Autodesk Inventor part; units mm, degrees
ref_plane "YZ Plane" through (0, 0, 0) normal (1, 0, 0) x (0, 1, 0)
ref_plane "XZ Plane" through (0, 0, 0) normal (0, 1, 0) x (-1, 0, 0)
ref_plane "XY Plane" through (0, 0, 0) normal (0, 0, 1) x (1, 0, 0)
sketch "Sketch1" plane through (0, 0, 0) normal (1, 0, 0) x (0, 1, 0)
  line L0 (10.2141, 17.9541) -> (-31.7859, 17.9541)
  line L1 (-31.7859, 17.9541) -> (-31.7859, -30.1559)
  line L2 (-31.7859, -30.1559) -> (10.2141, -30.1559)
  line L3 (10.2141, -30.1559) -> (10.2141, 17.9541)
  point P0 (0, 0)
  dimension "d0" = 42
  dimension "d1" = 48.11
extrude "BasePlate" add sketch "Sketch1" along normal blind 3
sketch "Sketch2" plane through (3, 0, 0) normal (1, 0, 0) x (0, 0, -1)
  point P0 (0, 0)
sketch "Sketch3" plane through (3, 0, 0) normal (1, 0, 0) x (0, 0, -1)
  line L0 (30.1559, 10.2141) -> (-17.9541, 10.2141)
  line L1 (-17.9541, -31.7859) -> (30.1559, -31.7859)
  line L2 (-17.9541, 10.2141) -> (30.1559, 10.2141)
  line L3 (30.1559, 10.2141) -> (30.1559, -31.7859)
  line L4 (30.1559, -31.7859) -> (-17.9541, -31.7859)
  line L5 (-17.9541, -31.7859) -> (-17.9541, 10.2141)
  line L6 (-15.5541, 8.2141) -> (27.7559, 8.2141)
  line L7 (27.7559, 8.2141) -> (27.7559, -29.3859)
  line L8 (27.7559, -29.3859) -> (-15.5541, -29.3859)
  line L9 (-15.5541, -29.3859) -> (-15.5541, 8.2141)
  point P0 (0, 0)
  point P1 (-17.9541, -10.7859)
  dimension "d4" = 2
  dimension "d5" = 2.4
  dimension "d6" = 2.4
  dimension "d7" = 2.4
extrude "Walls" add sketch "Sketch3" along normal blind 18.5
sketch "Sketch4" plane through (21.5, 0, 0) normal (1, 0, 0) x (0, 0, -1)
  line L0 (30.1559, 10.2141) -> (-17.9541, 10.2141)
  line L1 (-15.5541, 8.2141) -> (27.7559, 8.2141)
  line L2 (-4.1541, 10.2141) -> (5.2459, 10.2141)
  line L3 (5.2459, 10.2141) -> (5.2459, 8.2141)
  line L4 (5.2459, 8.2141) -> (-4.1541, 8.2141)
  line L5 (-4.1541, 8.2141) -> (-4.1541, 10.2141)
  line L6 (-17.9541, 10.2141) -> (-17.9541, -31.7859)
  point P0 (0, 0)
  point P1 (-4.1541, 9.2141)
  point P2 (5.2459, 10.2141)
  dimension "d10" = 9.4
  dimension "d11" = 13.8
extrude "USB-C" cut sketch "Sketch4" against normal blind 10.1
sketch "Sketch5" plane through (21.5, 0, 0) normal (1, 0, 0) x (0, 0, -1)
  line L0 (-17.9541, 10.2141) -> (-17.9541, -31.7859)
  line L1 (-15.5541, -29.3859) -> (-15.5541, 8.2141)
  line L2 (-17.9541, -4.8859) -> (-15.5541, -4.8859)
  line L3 (-15.5541, -4.8859) -> (-15.5541, 7.5141)
  line L4 (-15.5541, 7.5141) -> (-17.9541, 7.5141)
  line L5 (-17.9541, 7.5141) -> (-17.9541, -4.8859)
  line L6 (-4.1541, 10.2141) -> (-17.9541, 10.2141)
  point P0 (0, 0)
  point P1 (-16.7541, 7.5141)
  point P2 (-17.9541, 7.5141)
  point P3 (-15.5541, -4.8859)
  dimension "d14" = 12.4
  dimension "d15" = 2.7
extrude "PowerConnector1" cut sketch "Sketch5" against normal blind 15.5
sketch "Sketch6" plane through (6, 0, 0) normal (1, 0, 0) x (0, 0, -1)
  line L0 (-17.9541, 10.2141) -> (-17.9541, -31.7859)
  line L1 (-17.9541, -0.3859) -> (-15.5541, -0.3859)
  line L2 (-15.5541, -0.3859) -> (-15.5541, 1.6141)
  line L3 (-15.5541, 1.6141) -> (-17.9541, 1.6141)
  line L4 (-17.9541, 1.6141) -> (-17.9541, -0.3859)
  line L5 (-17.9541, 7.5141) -> (-15.5541, 7.5141)
  point P0 (0, 0)
  dimension "d18" = 2.4
  dimension "d19" = 2
  dimension "d20" = 5.9
extrude "PowerConnector2" cut sketch "Sketch6" against normal blind 2.5
sketch "Sketch8" plane through (21.5, 0, 0) normal (1, 0, 0) x (0, 0, -1)
  line L0 (-17.9541, 10.2141) -> (-17.9541, -31.7859)
  line L1 (-15.5541, 8.2141) -> (-15.5541, -29.3859)
  line L2 (-17.9541, -28.7859) -> (-15.5541, -28.7859)
  line L3 (-15.5541, -28.7859) -> (-15.5541, -15.1859)
  line L4 (-15.5541, -15.1859) -> (-17.9541, -15.1859)
  line L5 (-17.9541, -15.1859) -> (-17.9541, -28.7859)
  line L6 (-17.9541, -31.7859) -> (30.1559, -31.7859)
  point P0 (0, 0)
  dimension "d23" = 13.6
  dimension "d24" = 3
extrude "RJ-12" cut sketch "Sketch8" against normal blind 18.1
fillet "Fillet1" radius 0.5 4 edges at (10.75, 10.2141, 17.9541) (10.75, -31.7859, 17.9541) (10.75, 10.2141, -30.1559) (10.75, -31.7859, -30.1559)
sketch "Sketch9" plane through (0, 0, 0) normal (-1, 0, 0) x (0, 0, 1)
  line L0 (-24.5559, -25.4859) -> (-21.5559, -25.4859)
  line L1 (-21.5559, -25.4859) -> (-21.5559, -22.4859)
  line L2 (-21.5559, -22.4859) -> (-24.5559, -22.4859)
  line L3 (-24.5559, -22.4859) -> (-24.5559, -25.4859)
  line L4 (-30.1559, -31.2859) -> (-30.1559, 9.7141)
  line L5 (17.4541, -31.7859) -> (-29.6559, -31.7859)
  point P0 (0, 0)
  point P1 (-24.5559, -23.9859)
  dimension "d28" = 3
  dimension "d29" = 3
  dimension "d30" = 5.6
  dimension "d31" = 6.3
extrude "ZBButton" cut sketch "Sketch9" against normal blind 3
sketch "Sketch10" plane through (0, 0, 0) normal (-1, 0, 0) x (0, 0, 1)
  line L0 (-24.5559, 0.9141) -> (-21.5559, 0.9141)
  line L1 (-21.5559, 0.9141) -> (-21.5559, 3.9141)
  line L2 (-21.5559, 3.9141) -> (-24.5559, 3.9141)
  line L3 (-24.5559, 3.9141) -> (-24.5559, 0.9141)
  line L4 (-30.1559, -31.2859) -> (-30.1559, 9.7141)
  line L5 (-29.6559, 10.2141) -> (17.4541, 10.2141)
  point P0 (0, 0)
  point P1 (-24.5559, 2.4141)
  dimension "d34" = 3
  dimension "d35" = 3
  dimension "d36" = 5.6
  dimension "d37" = 6.3
extrude "ResetButton" cut sketch "Sketch10" against normal blind 3
sketch "Sketch11" plane through (3, 0, 0) normal (1, 0, 0) x (0, 0, -1)
  line L0 (25.5559, 4.9141) -> (20.5559, 4.9141)
  line L1 (20.5559, 4.9141) -> (20.5559, -0.0859)
  line L2 (20.5559, -0.0859) -> (25.5559, -0.0859)
  line L3 (25.5559, -0.0859) -> (25.5559, 4.9141)
  line L4 (21.5559, 3.9141) -> (24.5559, 3.9141)
  line L5 (24.5559, 3.9141) -> (24.5559, 0.9141)
  line L6 (25.5559, -21.4859) -> (20.5559, -21.4859)
  line L7 (20.5559, -21.4859) -> (20.5559, -26.4859)
  line L8 (20.5559, -26.4859) -> (25.5559, -26.4859)
  line L9 (25.5559, -26.4859) -> (25.5559, -21.4859)
  line L10 (24.5559, -22.4859) -> (24.5559, -25.4859)
  line L11 (21.5559, -22.4859) -> (24.5559, -22.4859)
  line L12 (24.5559, 0.9141) -> (21.5559, 0.9141)
  line L13 (24.5559, 3.9141) -> (21.5559, 3.9141)
  line L14 (21.5559, 3.9141) -> (21.5559, 0.9141)
  line L15 (21.5559, 0.9141) -> (24.5559, 0.9141)
  line L16 (24.5559, 0.9141) -> (24.5559, 3.9141)
  line L17 (21.5559, -25.4859) -> (21.5559, -22.4859)
  line L18 (24.5559, -22.4859) -> (21.5559, -22.4859)
  line L19 (21.5559, -22.4859) -> (21.5559, -25.4859)
  line L20 (21.5559, -25.4859) -> (24.5559, -25.4859)
  line L21 (24.5559, -25.4859) -> (24.5559, -22.4859)
  point P0 (0, 0)
  point P1 (23.0559, -22.4859)
  dimension "d40" = 5
  dimension "d41" = 5
  dimension "d42" = 1
  dimension "d43" = 1
  dimension "d44" = 5
  dimension "d45" = 5
  dimension "d46" = 1
  dimension "d47" = 1
extrude "ButtonFuehrung" add sketch "Sketch11" along normal blind 7
sketch "Sketch12" plane through (0, 0, 0) normal (-1, 0, 0) x (0, 0, 1)
  circle A0 centre (-16.9559, -27.1859) radius 0.75
  line L0 (17.4541, -31.7859) -> (-29.6559, -31.7859)
  line L1 (-30.1559, -31.2859) -> (-30.1559, 9.7141)
  point P0 (0, 0)
  dimension "d50" = 1.5
  dimension "d51" = 4.6
  dimension "d52" = 13.2
extrude "LED" cut sketch "Sketch12" against normal blind 3
sketch "Sketch13" plane through (11.4, 10.2141, 4.1541) normal (0, 1, 0) x (1, 0, 0)
  circle A0 centre (-3.4, 16.91) radius 3.2
  line L0 (-11.4, 33.81) -> (-11.4, -13.3)
  line L1 (10.1, 34.31) -> (-11.4, 34.31)
  point P0 (-11.4, 4.1541)
  dimension "d55" = 6.4
  dimension "d56" = 8
  dimension "d57" = 17.4
extrude "Antenna" cut sketch "Sketch13" against normal blind 2
sketch "Sketch14" plane through (3, 8.2141, -27.7559) normal (0, -1, 0) x (1, 0, 0)
  line L0 (17.5, 40.31) -> (16.5, 40.31)
  line L1 (16.5, 40.31) -> (16.5, 35.31)
  line L2 (16.5, 35.31) -> (17.5, 35.31)
  line L3 (17.5, 35.31) -> (17.5, 40.31)
  line L4 (18.5, 43.31) -> (18.5, 31.91)
  point P0 (-3, 27.7559)
  point P1 (17.5, 37.81)
  dimension "d60" = 1
  dimension "d61" = 5
  dimension "d62" = 1
  dimension "d63" = 5.5
extrude "Extrusion12" cut sketch "Sketch14" against normal blind 0.5
sketch "Sketch15" plane through (3, 8.2141, -27.7559) normal (0, -1, 0) x (1, 0, 0)
  line L0 (17.5, 13.5) -> (16.5, 13.5)
  line L1 (16.5, 13.5) -> (16.5, 8.5)
  line L2 (16.5, 8.5) -> (17.5, 8.5)
  line L3 (17.5, 8.5) -> (17.5, 13.5)
  line L4 (18.5, 22.51) -> (18.5, 0)
  line L5 (0, 0) -> (18.5, 0)
  point P0 (-3, 27.7559)
  point P1 (17.5, 11)
  dimension "d66" = 1
  dimension "d67" = 5
  dimension "d68" = 1
  dimension "d69" = 11
extrude "Extrusion13" cut sketch "Sketch15" against normal blind 0.5
sketch "Sketch16" plane through (3, -29.3859, 15.5541) normal (0, 1, 0) x (1, 0, 0)
  line L0 (17.5, 8) -> (16.5, 8)
  line L1 (16.5, 8) -> (16.5, 3)
  line L2 (16.5, 3) -> (17.5, 3)
  line L3 (17.5, 3) -> (17.5, 8)
  line L4 (18.5, 43.31) -> (18.5, 0)
  line L5 (0, 0) -> (18.5, 0)
  point P0 (-3, 15.5541)
  point P1 (17.5, 5.5)
  dimension "d72" = 1
  dimension "d73" = 5
  dimension "d74" = 1
  dimension "d75" = 5.5
extrude "Extrusion14" cut sketch "Sketch16" against normal blind 0.5
sketch "Sketch17" plane through (3, -29.3859, 15.5541) normal (0, 1, 0) x (1, 0, 0)
  line L0 (17.5, 34.81) -> (16.5, 34.81)
  line L1 (16.5, 34.81) -> (16.5, 29.81)
  line L2 (16.5, 29.81) -> (17.5, 29.81)
  line L3 (17.5, 29.81) -> (17.5, 34.81)
  line L4 (18.5, 43.31) -> (18.5, 0)
  line L5 (0, 43.31) -> (18.5, 43.31)
  point P0 (-3, 15.5541)
  point P1 (17.5, 32.31)
  dimension "d78" = 1
  dimension "d79" = 5
  dimension "d80" = 1
  dimension "d81" = 11
extrude "Extrusion15" cut sketch "Sketch17" against normal blind 0.5
equation "\"BendRadius\" = Thickness"
equation "\"BendReliefWidth\" = Thickness"
equation "\"BendReliefDepth\" = 0.5 * Thickness"
equation "\"CornerReliefSize\" = 4 * Thickness"
equation "\"MinimumRemnant\" = 2 * Thickness"
equation "\"TransitionRadius\" = BendRadius"
equation "\"JacobiRadiusSize\" = BendRadius"
equation "\"GapSize\" = Thickness"
properties part number "Enclosure_Top_v2"
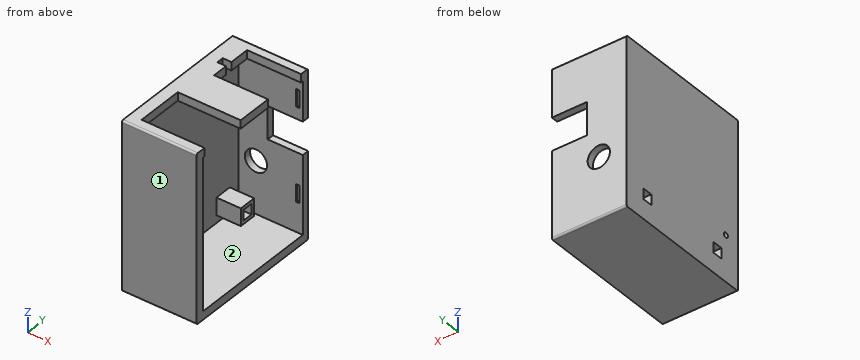
Can you work these out from the model? Positions are in its coordinate system, mm. Face numbers are marked on the shaded views. A direction names the side the tool comes from. Round coordinates to 2 decimals unless told otherwise and drop trailing zeros. Order: outer loops, then holes, each group sorted by start corner. A loop starts at its lowest first (then second) coordinate and runs counter-clockwise, first axis right, second up. Notation, with made-up numbers: (72, -9.75) -> (102, -9.75) arc R21 cw to (102, 23.25) -> close; hole circle Ø3 at (-16.5, 61). An arc over 180 degrees is marked (long way). Return JSON: item names as keys, results as strings. Group by question number.
1. Will these pins go through, and if not, where does the flat tip stop? pin 1 (12 mm diameter, centred on y = -5, z = 1.5, fed in from +X); pin 2 (2.5 mm diameter, centred on y = -25, z = -24.5, fed in from +X); pin 3 (3 mm diameter, centred on x = 12, y = -2, fed in from +Z).
2. Which directions (+Z, -Z, +X, -X, +Y, -Y) give clear straight access to the entire face, cutting with the end or side of a thin tool? Please do the marked faces 1 and 2.
3. I need wall thicknesses on line 1 (Y direction, x = 9, z = -24.5); line 2 (Z direction, x = 19.25, y = -9.5); line 3 (Z direction, x = 8, y = 9.1). Which ranges of each line are inside material? Lowest first, please. Write a range as [from, to].
4. If we section it at C-C, the plane x = 8: Count the separate pieces of the cut face and the enclosed holes in it, then the cut area to 3 significant figures.
5. If we section it at B-B, the plane z = -4: Write out the boundary of the cut face in (x, y).
6. If we section it at D-D, the plane y = -16: Write out the boundary of the cut face in (x, z), then the cut area to 3 significant figures.
7. If we section it at A-A, the plane y = -24: Write out the boundary of the cut face in (x, z), then the cut area to 3 significant figures.
Output values:
{
 "1": {"pin 1": "x = 3", "pin 2": "x = 10", "pin 3": "z = -27.76"},
 "2": {"face 1": "+Z, -Z, +X, -X, -Y", "face 2": "+X"},
 "3": {"line 1": "[-31.79, -29.39], [-26.49, -25.49], [-22.49, -21.49], [-0.09, 0.91], [3.91, 4.91], [8.21, 10.21]", "line 2": "[-30.16, -27.76], [15.55, 17.95]", "line 3": "[-30.16, -15.96], [-9.56, 17.95]"},
 "4": {"separate pieces": "5", "enclosed holes": "2", "area": "349 mm²"},
 "5": {"outline": "(0, -31.79) -> (21.5, -31.79) -> (21.5, -29.39) -> (3, -29.39) -> (3, 8.21) -> (11.4, 8.21) -> (11.4, 10.21) -> (0, 10.21) -> close"},
 "6": {"outline": "(0, -30.16) -> (21.5, -30.16) -> (21.5, -27.76) -> (3, -27.76) -> (3, 15.55) -> (3.4, 15.55) -> (3.4, 17.95) -> (0, 17.95) -> close", "area": "190 mm²"},
 "7": {"outline": "(0, -30.16) -> (21.5, -30.16) -> (21.5, -27.76) -> (3, -27.76) -> (3, -25.56) -> (10, -25.56) -> (10, -24.56) -> (0, -24.56) -> close; (0, -21.56) -> (10, -21.56) -> (10, -20.56) -> (3, -20.56) -> (3, 15.55) -> (3.4, 15.55) -> (3.4, 17.95) -> (0, 17.95) -> close", "area": "195 mm²"}
}
